Verification items for the finished model (mm, model axes). Face numbers are marked on the shaded views. A direction names the side the tool comes from. Give positions to 0.01 mm unless a question says otherwise; leave off trailing zeros. Loops run counter-clockwise (first coordinate to the right, second up) from the corner with the lowest first, then second, coordinate; pieces in that order, holes last. Notation, with made-up numbers: (42, 84.25) -> (73, 84.25) arc R29 ccw to (73, 119.25) -> close; hole circle Ø8 at (74.25, 68.5). An arc over 180 degrees is marked (long way). Answer in a Markdown table with one row per item. Add a question column.
Q1. Material ranges on probe 1 along X at (y, z) = (5, 0); probe 2 along X at (y, z) = (6.5, 0), recorded low to high.
Q2. Section check B-B on x = 0. Enter the section's corners in (y, z).
Q3. Gauge pin test, flat ends, axial feed: P1, Ø2, axis at x = 6.5, z = -7, coming from the -Y side; P2, Ø4, axis at x = -1.5, y = 2.5, coming from the -Z side; P3, Ø7.5, axis at x = 0, z = 0, coming from the -Y side; P4, Ø2, axis at y = 4.5, z = 9.5, coming from the +X side. Record the tip position at first contact, or that the pin passes through.
Q4. Section check C-C on y = 4.5. Enter the section's corners in (x, z).
Q5. Section check D-D on y = 2.75. Enter the section's corners in (x, z), and give its area (3 significant figures).
Q6. Release check for a two-part mould opening along Z. For the marked faces 1, 2 and 3 record: pulls with the +Z half, pulls with the -Z half, needs draft (parallel to the pull), parting line crosses it, or undercut.
Q7. Section check A-A on z = 0. Enter the section's corners in (x, y).
Q8. Set-up check for the marked faces 4 and 5: record each of +Z, -Z, +X, -X, +Y, -Y from which the full face is reachable in a straight line by a thin tool's end or side.
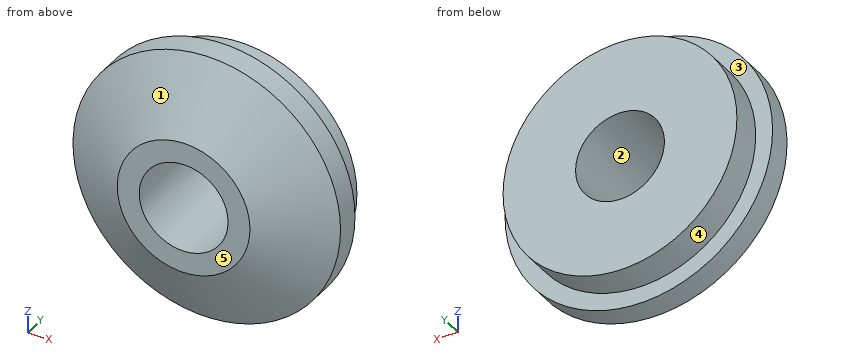
```python
from build123d import *

# Parameters (mm, degrees)
SKETCH1_R         = 12.7
EXTRUDE1_DEPTH    = 9
SKETCH2_R         = 4.2164
EXTRUDE2_DEPTH    = 25.4
SKETCH3_OUTSIDE_W = 34.806
SKETCH3_OUTSIDE_H = 34.806
SKETCH3_OUTSIDE_R = 11.1
EXTRUDE3_DEPTH    = 3


with BuildPart() as part:
    # Sketch1 → Extrude1 (new body)
    with BuildSketch(Plane(origin=(0, 0, 0), x_dir=(1, 0, 0), z_dir=(0, 1, 0))):
        Circle(SKETCH1_R)
    extrude(amount=EXTRUDE1_DEPTH)

    # Sketch2 → Extrude2 (cut)
    with BuildSketch(Plane(origin=(0, 0, 0), x_dir=(1, 0, 0), z_dir=(0, 1, 0))):
        Circle(SKETCH2_R)
    extrude(amount=EXTRUDE2_DEPTH, mode=Mode.SUBTRACT)

    # Sketch3 outside → Extrude3 (cut)
    with BuildSketch(Plane(origin=(0, 9, 0), x_dir=(1, 0, 0), z_dir=(0, 1, 0))):
        Rectangle(SKETCH3_OUTSIDE_W, SKETCH3_OUTSIDE_H)
        Circle(SKETCH3_OUTSIDE_R, mode=Mode.SUBTRACT)
    extrude(amount=-EXTRUDE3_DEPTH, mode=Mode.SUBTRACT)

    # Sketch6 → Cut-Revolve1 (revolve, cut)
    with BuildSketch(Plane(origin=(0, 0, 0), x_dir=(0, 0, -1), z_dir=(1, 0, 0))):
        Polygon((-1.103847577, -3), (-15, 5.022947342), (-15, -3), align=None)
    revolve(axis=Axis((0, 0, 0), (0, -1, 0)), mode=Mode.SUBTRACT)


solid = part.part
```
Taken from the geometry:
| question | item | result |
|---|---|---|
| 1 | probe 1 | x = -12.7 to -4.22, 4.22 to 12.7 |
| 1 | probe 2 | x = -11.1 to -4.22, 4.22 to 11.1 |
| 2 | outline | (0, -6.3) -> (3.7, -12.7) -> (6, -12.7) -> (6, -11.1) -> (9, -11.1) -> (9, -4.22) -> (0, -4.22) -> close; (0, 4.22) -> (9, 4.22) -> (9, 11.1) -> (6, 11.1) -> (6, 12.7) -> (3.7, 12.7) -> (0, 6.3) -> close |
| 3 | P1 | stops at y = 1.3 |
| 3 | P2 | stops at z = -12.7 |
| 3 | P3 | passes through |
| 3 | P4 | stops at x = 9.44 |
| 4 | outline | circle Ø25.4 at (0, 0); hole circle Ø8.43 at (0, 0) |
| 5 | outline | circle Ø22.13 at (0, 0); hole circle Ø8.43 at (0, 0) |
| 5 | area | 329 mm² |
| 6 | face 1 | parting line crosses it |
| 6 | face 2 | undercut |
| 6 | face 3 | needs draft |
| 7 | outline | (-12.7, 3.7) -> (-6.3, 0) -> (-4.22, 0) -> (-4.22, 9) -> (-11.1, 9) -> (-11.1, 6) -> (-12.7, 6) -> close; (4.22, 0) -> (6.3, 0) -> (12.7, 3.7) -> (12.7, 6) -> (11.1, 6) -> (11.1, 9) -> (4.22, 9) -> close |
| 8 | face 4 | +Y |
| 8 | face 5 | +Z, -Z, +X, -X, -Y |
